Geometry: see drawing. Coordinates: mm, zero at the bounding-box minimum. A direction names the side the tool comes from. Give positions to 0.01 mm unless a question says otherwise; leave off trailing zeros. Loops run counter-clockwise (first coordinate to the right, second up) from the corner with the lowest first, then second, coordinate; pieces in that order, holes last. Notation, with made-up numbers: M 41,57 L 87,57 A29 cw 87,78 Z; hole C -13.75,-20 d5. An arc over 180 degrees is marked long. Use CSV: the item, a comma, the result in double quotes. Start each with the question number.
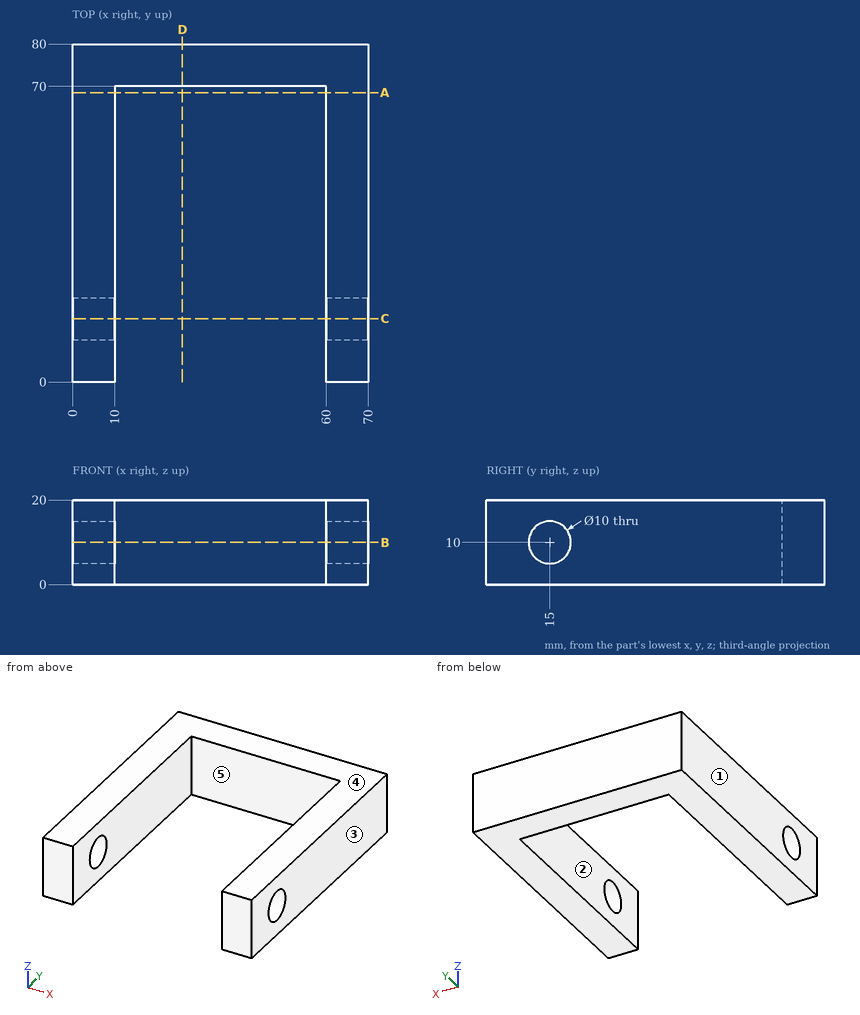
Item 1: Section D-D (x = 26). Output: boundary loops of the cut face in (y, z), then the cut area to 3 significant figures.
Item 2: Set-up query: the marked faces 1 and 2. Return all of +Z, -Z, +X, -X, +Y, -Y with unobstructed straight access to the full face (end or side cutting, diameter ignored); none if empty.
Item 3: Section B-B (z = 10). Output: boundary loops of the cut face in (x, y), then the cut area to 3 significant figures.
Item 4: Section A-A (y = 68.5). Output: boundary loops of the cut face in (x, z).
Item 5: First-contact query: pin 1 Ø5 at (x, z) = (57, 11.5) entering from -Y. Flat tip, straight axial feed; report the tip coordinate or a pass-through.
Item 6: Mould query, pull axis X, two halves, no side actions, for the marked faces 3, 4 and 5. Classes: +X half, -X half, draft (parallel to the pull), parting line (faces both ways), or undercut.
Item 7: Material intervals for line 1 (X direction, y = 28, z = 14.5); line 2 (Y direction, x = 2.25, z = 10); line 3 (Y direction, x = 53, z = 12.25), sorted ascending.
Item 8: Section C-C (y = 15). Output: boundary loops of the cut face in (x, z), then the cut area to 3 significant figures.
Recorded:
1,outline,"M 70,0 L 80,0 L 80,20 L 70,20 Z"
1,area,"200 mm²"
2,face 1,"+Z, -Z, -X, +Y, -Y"
2,face 2,"+Z, -Z, -Y"
3,outline,"M 0,0 L 10,0 L 10,10 L 0,10 Z; M 0,20 L 10,20 L 10,70 L 60,70 L 60,20 L 70,20 L 70,80 L 0,80 Z; M 60,0 L 70,0 L 70,10 L 60,10 Z"
3,area,"1,900 mm²"
4,outline,"M 0,0 L 10,0 L 10,20 L 0,20 Z; M 60,0 L 70,0 L 70,20 L 60,20 Z"
5,pin 1,"y = 70"
6,face 3,"+X half"
6,face 4,"draft"
6,face 5,"undercut"
7,line 1,"0 to 10, 60 to 70"
7,line 2,"0 to 10, 20 to 80"
7,line 3,"70 to 80"
8,outline,"M 0,0 L 10,0 L 10,5 L 0,5 Z; M 0,15 L 10,15 L 10,20 L 0,20 Z; M 60,0 L 70,0 L 70,5 L 60,5 Z; M 60,15 L 70,15 L 70,20 L 60,20 Z"
8,area,"200 mm²"
